from build123d import *

# Parameters (mm, degrees)
SKETCH004_W             = 35.6
SKETCH004_H             = 11.6
PAD003_DEPTH            = 0.8
SKETCH005_W             = 35.6
SKETCH005_H             = 11.6
SKETCH005_W_2           = 34
SKETCH005_H_2           = 10
PAD004_DEPTH            = 55.8
SKETCH006_W             = 4
SKETCH006_H             = 12
POCKET001_DEPTH         = 5.8
BODY002_PLACEMENT_ANGLE = 90


with BuildPart() as part:
    # Sketch004 → Pad003 (new body)
    with BuildSketch(Plane.XY):
        Rectangle(SKETCH004_W, SKETCH004_H)
    extrude(amount=PAD003_DEPTH)

    # Sketch005 → Pad004 (join)
    with BuildSketch(Plane.XY):
        Rectangle(SKETCH005_W, SKETCH005_H)
        Rectangle(SKETCH005_W_2, SKETCH005_H_2, mode=Mode.SUBTRACT)
    extrude(amount=PAD004_DEPTH)

    # Sketch006 → Pocket001 (cut, symmetric)
    with BuildSketch(Plane.XZ):
        with Locations((-15.8, 49.8)):
            Rectangle(SKETCH006_W, SKETCH006_H)
    extrude(amount=POCKET001_DEPTH, both=True, mode=Mode.SUBTRACT)


with BuildPart() as part_1:
    # Body002 placement: moved
    add(part.part.moved(Location((17.4, 28, 57.1))).rotate(Axis((17.4, 28, 57.1), (1, 0, 0)), BODY002_PLACEMENT_ANGLE))


solid = part_1.part
Read the model definition and answer for the solid it produces. Units are mm, in the model's axes. A direction names the side the tool comes from. Round coordinates to 2 decimals unless told otherwise and drop trailing zeros. Order: outer loops, then holes, each group sorted by start corner. A loop starts at its lowest first (then second) coordinate and runs counter-clockwise, first axis right, second up. Notation, with made-up numbers: (85, 16.25) - (123, 16.25) arc R28 ccw to (123, 37.25) - close; hole circle Ø8 at (6, 15). An arc over 180 degrees is marked (long way). Use one line per item in the form item = value. Start each with the question number.
(1) The part is cut by section B-B (x = 6). Give the vertices of the cut face in (y, z).
(2) For faces 4 (the face through (35.2, 0, 57)), 5 (the face through (34.4, 0, 57)), 6 (the face through (0, -15.8, 57)), determine the directions among +Z, -Z, +X, -X, +Y, -Y from which every point of the face is accessible in a straight line to the end or side of a thin tool.
(3) The part is cut by section A-A (y = 7). Give the vertices of the cut face in (x, z).
(4) Determine the mould class of faces 1 (the face through (-0.4, 6, 57)), 2 (the face through (17, 0, 51.3)), 3 (the face through (17, 0, 52.1)) for opening direction Z: +Z half, -Z half, draft (parallel to the pull), parting line (faces both ways), or undercut.
(5) Find the intervals of material crossed by line 1 along X through (y, z) = (-5, 53); line 2 along Z through (x, y) = (29.5, -11.5); line 3 along X through (y, z) = (-21, 56.25), in increasing order. Write a range as from..to.
(6) Flat-ended cylindrical pins translate along their axes: pin 1 Ø5 at (x, z) = (11.5, 57) entering from -Y; pin 2 Ø2 at (x, z) = (1, 60) entering from -Y; pin 3 Ø0.9 at (y, z) = (-19.5, 51.5) entering from -X. Find the tip coordinate at first contact, or state that the pin passes through.
(7) The part is cut by section C-C (z = 60.25). Give the vertices of the cut face in (x, y), then the cut area to 3 significant figures.
Checked values:
q1.outline = (-27.8, 51.3) - (28, 51.3) - (28, 62.9) - (-27.8, 62.9) - (-27.8, 62.1) - (27.2, 62.1) - (27.2, 52.1) - (-27.8, 52.1) - close
q2.face_4 = +Z, -Z, +X, +Y, -Y
q2.face_5 = -Y
q2.face_6 = +Z, -Z, -X, -Y
q3.outline = (-0.4, 51.3) - (35.2, 51.3) - (35.2, 62.9) - (-0.4, 62.9) - close; hole (0.4, 52.1) - (34.4, 52.1) - (34.4, 62.1) - (0.4, 62.1) - close
q4.face_1 = draft
q4.face_2 = -Z half
q4.face_3 = undercut
q5.line_1 = -0.4..0.4, 34.4..35.2
q5.line_2 = 51.3..52.1, 62.1..62.9
q5.line_3 = 34.4..35.2
q6.pin_1 = 27.2
q6.pin_2 = -15.8
q6.pin_3 = 3.6
q7.outline = (-0.4, -15.8) - (0.4, -15.8) - (0.4, 27.2) - (34.4, 27.2) - (34.4, -27.8) - (35.2, -27.8) - (35.2, 28) - (-0.4, 28) - close
q7.area = 107 mm^2
